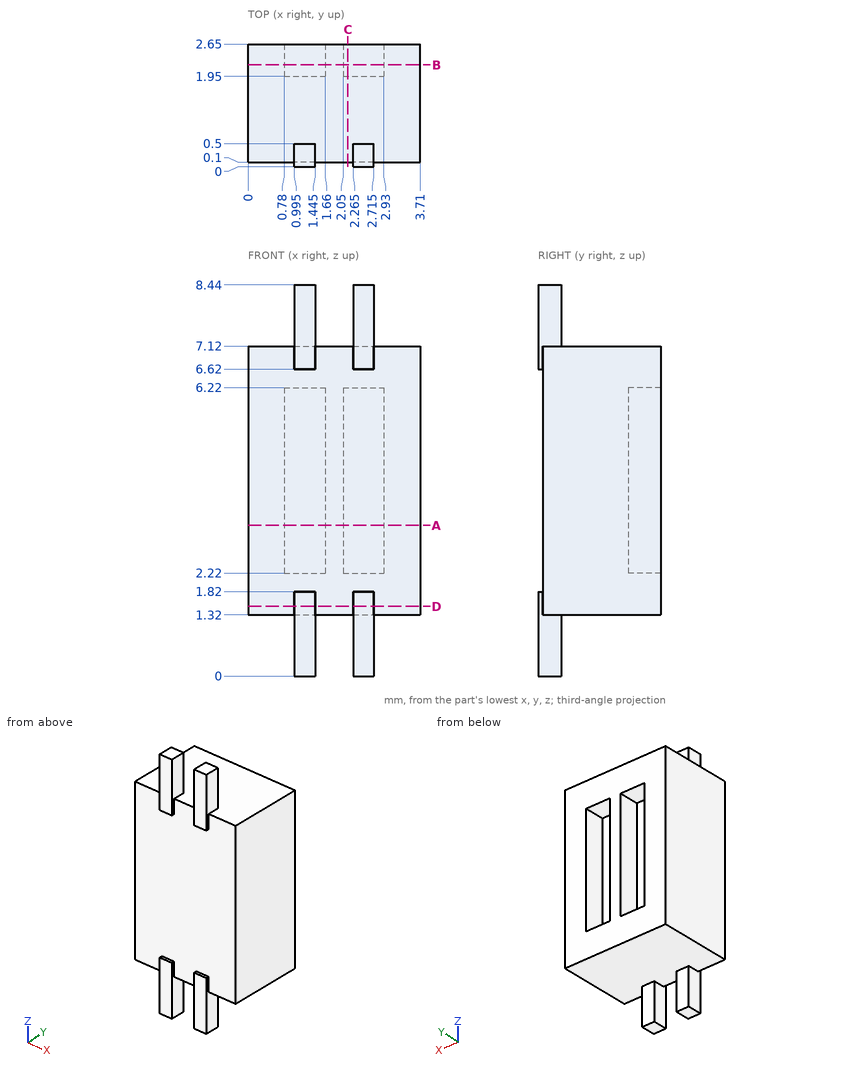
Drawing for the job (mm, zero at the part's lowest x, y, z). Round coordinates to 2 decimals unless told otherwise and drop trailing zeros. Order: outer loops, then holes, each group sorted by start corner. A loop starts at its lowest first (then second) coordinate and runs counter-clockwise, first axis right, second up.
Item 1: Saw through at B-B on y = 2.2. Write the cut outline in (x, z), then the cut area to 3 significant figures.
Item 2: Probe line 1 along X through (y, z) = (2.4, 5); line 2 along X through (y, z) = (0.2, 0.5) (3 decimals); line 3 along Z through (x, y) = (2.4, 1.35). List the from-to ranges inside material, lowest first.
Item 3: Saw through at A-A on z = 3.25. Write the cut outline in (x, y), then the cut area to 3 significant figures.
Item 4: Pin check, flat tips, straight feed: pin 1 (0.8 mm diameter, centred on y = 2, z = 5, fed in from -X); pin 2 (0.5 mm diameter, centred on x = 2.5, z = 7.5, fed in from +Y); pin 3 (0.8 mm diameter, centred on x = 2.5, y = 2.5, fed in from +Z); pin 4 (0.6 mm diameter, centred on x = 1, y = 2, fed in from -Z). Stop position of each tip, or through.
Item 5: Saw through at C-C on x = 2.15. Write the cut outline in (y, z), then the cut area to 3 significant figures.
Item 6: Saw through at D-D on z = 1.5. Write the cut outline in (x, y) (3 decimals), then the cut area to 3 significant figures.
Reported:
1. outline: (0, 1.32) - (3.71, 1.32) - (3.71, 7.12) - (0, 7.12) - close; hole (0.78, 2.22) - (1.66, 2.22) - (1.66, 6.22) - (0.78, 6.22) - close; hole (2.05, 2.22) - (2.93, 2.22) - (2.93, 6.22) - (2.05, 6.22) - close
1. area: 14.5 mm2
2. line 1: x = 0 to 0.78, 1.66 to 2.05, 2.93 to 3.71
2. line 2: x = 0.995 to 1.445, 2.265 to 2.715
2. line 3: z = 1.32 to 7.12
3. outline: (0, 0.1) - (3.71, 0.1) - (3.71, 2.65) - (2.93, 2.65) - (2.93, 1.95) - (2.05, 1.95) - (2.05, 2.65) - (1.66, 2.65) - (1.66, 1.95) - (0.78, 1.95) - (0.78, 2.65) - (0, 2.65) - close
3. area: 8.23 mm2
4. pin 1: stops at x = 0
4. pin 2: stops at y = 0.5
4. pin 3: stops at z = 7.12
4. pin 4: stops at z = 1.32
5. outline: (0.1, 1.32) - (2.65, 1.32) - (2.65, 2.22) - (1.95, 2.22) - (1.95, 6.22) - (2.65, 6.22) - (2.65, 7.12) - (0.1, 7.12) - close
5. area: 12.0 mm2
6. outline: (0, 0.1) - (0.995, 0.1) - (0.995, 0) - (1.445, 0) - (1.445, 0.1) - (2.265, 0.1) - (2.265, 0) - (2.715, 0) - (2.715, 0.1) - (3.71, 0.1) - (3.71, 2.65) - (0, 2.65) - close
6. area: 9.55 mm2
